Model file for the job. Use its own axes, mm. Coordinates: 2 decimals unless noted, no trailing zeros. Order: outer loops, then holes, each group sorted by start corner. A loop starts at its lowest first (then second) coordinate and runs counter-clockwise, first axis right, second up. Notation, with made-up numbers: M 57,-12 L 97,-12 A11 ccw 97,1 Z; hole C 23.5,7 d5. An arc over 180 degrees is marked long. Return JSON: item names as keys, results as strings.
Autodesk Inventor part; units mm, degrees
ref_plane "YZ Plane" through (0, 0, 0) normal (1, 0, 0) x (0, 1, 0)
ref_plane "XZ Plane" through (0, 0, 0) normal (0, 1, 0) x (-1, 0, 0)
ref_plane "XY Plane" through (0, 0, 0) normal (0, 0, 1) x (1, 0, 0)
sketch "Sketch1" plane through (0, 0, 0) normal (0, 1, 0) x (-1, 0, 0)
  circle A0 centre (0, 0) radius 13
  dimension "d0" = 26
extrude "Extrusion1" add sketch "Sketch1" along normal blind 1
sketch "Sketch2" plane through (0, 1, 0) normal (0, 1, 0) x (1, 0, 0)
  circle A0 centre (0, 0) radius 5.25
  dimension "d3" = 10.5
extrude "Extrusion2" add sketch "Sketch2" along normal blind 2
sketch "Sketch3" plane through (0, 1, 0) normal (0, 1, 0) x (1, 0, 0)
  circle A0 centre (0, 0) radius 5.25
  circle A1 centre (0, 0) radius 13
  circle A2 centre (0, 0) radius 10.5
  dimension "d6" = 21
extrude "Extrusion3" cut sketch "Sketch3" against normal blind 2 contours A1
properties part number "plastic washer for washer magnet bases"
Item 1: Drop a flat-ended pin along its axis: pin 1 Ø3 at (x, z) = (0.5, -1) entering from -Y. Give the stop position or say it passes through.
Check result:
{"pin 1": "stops at y = 0"}
Item 2: Pull direction Z, two halves, no side cores. Call faces 1 (the cylindrical face through (5, 2, 1.6)), 2 (the flat face through (2.5, 1, 4.8)): +Z half, -Z half, draft (parallel to the pull), parting line (faces both ways), or undercut.
Check result:
{"face 1": "parting line", "face 2": "draft"}
Item 3: Saw through at C-C (y = 2.3). Write the cut outline in (x, z), and give its area (3 significant figures).
Check result:
{"outline": "C 0,0 d10.5", "area": "86.6 mm2"}
Item 4: Saw through at D-D (y = 0.45). Write the cut outline in (x, z).
Check result:
{"outline": "C 0,0 d21"}
Item 5: Saw through at A-A (x = 0). Write the cut outline in (y, z).
Check result:
{"outline": "M 0,-10.5 L 1,-10.5 L 1,-5.25 L 3,-5.25 L 3,5.25 L 1,5.25 L 1,10.5 L 0,10.5 Z"}
Item 6: Saw through at B-B (z = 0). Write the cut outline in (x, y), and give its area (3 significant figures).
Check result:
{"outline": "M -10.5,0 L 10.5,0 L 10.5,1 L 5.25,1 L 5.25,3 L -5.25,3 L -5.25,1 L -10.5,1 Z", "area": "42.0 mm2"}
Item 7: Wall check: line 1 (Y direction, x = -0.5, z = -7.5); line 2 (Z direction, x = 5.75, y = 0.65); line 3 (X direction, y = 0.4, z = 8). Give the ranges that are in metal, low to high.
Check result:
{"line 1": "y = 0 to 1", "line 2": "z = -8.79 to 8.79", "line 3": "x = -6.8 to 6.8"}
